Here's how the part is built. I have some questions about the finished solid (model axes, mm). Face numbers are marked on the shaded views. A direction names the side the tool comes from. Give positions to 0.01 mm unless a question says otherwise; leave off trailing zeros. Loops run counter-clockwise (first coordinate to the right, second up) from the corner with the lowest first, then second, coordinate; pieces in that order, holes last. Notation, with made-up numbers: M 23.25,-27.5 L 61.25,-27.5 A17 ccw 61.25,-3.5 Z; hole C 88.5,-19.5 d3. An arc over 180 degrees is marked long. Answer as CSV lines item,"result". Start each with the question number.
Item 1: I want a section at B-B on z = 1.4. List the corners of the cut face in (x, y) for me.
Item 2: I want a section at A-A on x = 20. List the corners of the cut face in (y, z) for me.
Item 3: If I drill on line 1 along X through (y, z) = (7.5, 0.25); line 2 along X through (y, z) = (6, 3); line 3 along Y through (x, z) = (28, 0.3), over which ranges is the centre line in solid material (lowest first)? Write a range as from..to.
Item 4: I want a section at D-D on z = 3.75. List the corners of the cut face in (x, y) for me, plus the area to 3 significant figures.
Item 5: For the marked faces 1, 2 and 3, which set-ups out of +Z, -Z, +X, -X, +Y, -Y let a thin tool reach every point of the face, with its end or its side?
Item 6: Will these pins go through, and if not, where does the flat tip stop? P1, Ø0.9, axis at x = 12.5, y = 33.5, coming from the -Z side; P2, Ø5, axis at x = 9.5, y = 10.5, coming from the -Z side; P3, Ø12.5, axis at x = 10, y = 7.5, coming from the +Z side.
Item 7: I want a section at C-C on x = 10. List the corners of the cut face in (y, z) for me.
Item 8: If we mould it in two halves opening along Y, with no side actions, what happens to the marked faces 4, 5 and 6? For each: released by +Y, released by -Y, zero draft, split by the parting line, or undercut.
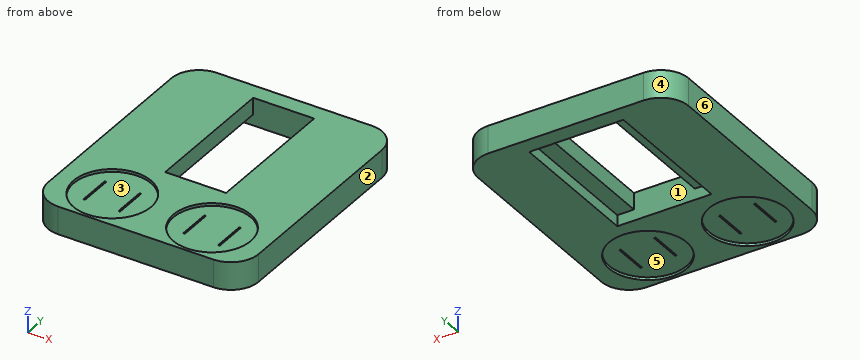
from build123d import *

# Parameters (mm, degrees)
F0_W      = 38
F0_H      = 45
F1_DEPTH  = 5
F2_R      = 7
F3_DEPTH  = 0.5
F2_W      = 5.5
F2_H      = 25
F4_DEPTH  = 5.001
F5_W      = 3
F5_H      = 25
F6_DEPTH  = 2
F7_W      = 0.3
F7_H      = 6
F8_DEPTH  = 5
F9_R      = 7
F10_DEPTH = 0.5
F11_R     = 5


with BuildPart() as f1:
    # F0 (on Top) → F1 (new body)
    with BuildSketch(Plane.XY):
        with Locations((19, 22.5)):
            Rectangle(F0_W, F0_H)
    extrude(amount=F1_DEPTH)

    # F2 (on face) → F3 (cut)
    with BuildSketch(Plane.XY.offset(5)):
        with Locations((10, 7.5)):
            Circle(F2_R)
        with Locations((28, 7.5)):
            Circle(F2_R)
    extrude(amount=-F3_DEPTH, mode=Mode.SUBTRACT)

    # F2 (on face) → F4 (cut, through all)
    with BuildSketch(Plane.XY.offset(5)):
        with Locations((16.25, 29.5)):
            Rectangle(F2_W, F2_H)
        with Locations((21.75, 29.5)):
            Rectangle(F2_W, F2_H)
    extrude(amount=-F4_DEPTH, mode=Mode.SUBTRACT)

    # F5 (on face) → F6 (cut)
    with BuildSketch(Plane(origin=(0, 0, 0), x_dir=(1, 0, 0), z_dir=(0, 0, -1))):
        with Locations((26, -29.5)):
            Rectangle(F5_W, F5_H)
        with Locations((12, -29.5)):
            Rectangle(F5_W, F5_H)
    extrude(amount=-F6_DEPTH, mode=Mode.SUBTRACT)

    # F7 (on face) → F8 (cut)
    with BuildSketch(Plane.XY.offset(4.5)):
        with Locations((6.85, 7.5)):
            Rectangle(F7_W, F7_H)
        with Locations((13.15, 7.5)):
            Rectangle(F7_W, F7_H)
        with Locations((24.85, 7.5)):
            Rectangle(F7_W, F7_H)
        with Locations((31.15, 7.5)):
            Rectangle(F7_W, F7_H)
    extrude(amount=-F8_DEPTH, mode=Mode.SUBTRACT)

    # F9 (on face) → F10 (cut)
    with BuildSketch(Plane(origin=(0, 0, 0), x_dir=(1, 0, 0), z_dir=(0, 0, -1))):
        with Locations((28, -7.5)):
            Circle(F9_R)
        with Locations((10, -7.5)):
            Circle(F9_R)
    extrude(amount=-F10_DEPTH, mode=Mode.SUBTRACT)

    # F11
    f11_edges = [f1.edges().sort_by_distance(p)[0] for p in [
        (0, 0, 2.5),
        (38, 0, 2.5),
        (38, 45, 2.5),
        (0, 45, 2.5),
    ]]
    fillet(f11_edges, radius=F11_R)


solid = f1.part
Result:
1,outline,"M 0,5 A5 ccw 5,0 L 33,0 A5 ccw 38,5 L 38,40 A5 ccw 33,45 L 5,45 A5 ccw 0,40 Z; hole M 6.7,4.5 L 7,4.5 L 7,10.5 L 6.7,10.5 Z; hole M 10.5,17 L 27.5,17 L 27.5,42 L 10.5,42 Z; hole M 13,4.5 L 13.3,4.5 L 13.3,10.5 L 13,10.5 Z; hole M 24.7,4.5 L 25,4.5 L 25,10.5 L 24.7,10.5 Z; hole M 31,4.5 L 31.3,4.5 L 31.3,10.5 L 31,10.5 Z"
2,outline,"M 0,0 L 17,0 L 17,5 L 0,5 Z; M 42,0 L 45,0 L 45,5 L 42,5 Z"
3,line 1,"0..3, 17..21, 35..38"
3,line 2,"0..6.7, 7..13, 13.3..24.7, 25..31, 31.3..38"
3,line 3,"0..0.5, 14.5..45"
4,outline,"M 0,5 A5 ccw 5,0 L 33,0 A5 ccw 38,5 L 38,40 A5 ccw 33,45 L 5,45 A5 ccw 0,40 Z; hole M 6.7,4.5 L 7,4.5 L 7,10.5 L 6.7,10.5 Z; hole M 13,4.5 L 13.3,4.5 L 13.3,10.5 L 13,10.5 Z; hole M 13.5,17 L 24.5,17 L 24.5,42 L 13.5,42 Z; hole M 24.7,4.5 L 25,4.5 L 25,10.5 L 24.7,10.5 Z; hole M 31,4.5 L 31.3,4.5 L 31.3,10.5 L 31,10.5 Z"
4,area,"1,410 mm^2"
5,face 1,"-Z"
5,face 2,"+Z, -Z, +X, +Y, -Y"
5,face 3,"+Z"
6,P1,"z = 2"
6,P2,"z = 0.5"
6,P3,"z = 4.5"
7,outline,"M 0,0 L 0.5,0 L 0.5,0.5 L 14.5,0.5 L 14.5,0 L 45,0 L 45,5 L 14.5,5 L 14.5,4.5 L 0.5,4.5 L 0.5,5 L 0,5 Z"
8,face 4,"released by +Y"
8,face 5,"undercut"
8,face 6,"zero draft"
